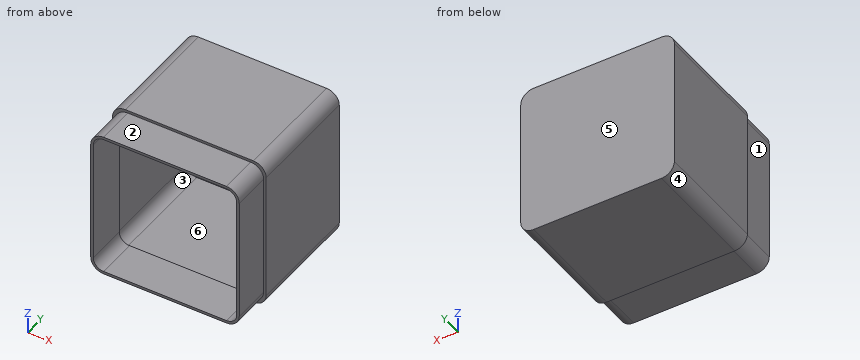
from build123d import *

# Parameters (mm, degrees)
F0_W     = 30.48
F0_H     = 30.48
F1_DEPTH = 22.86
F2_W     = 29.464
F2_H     = 29.464
F3_DEPTH = 7.62
F4_R     = 2.54
F5_T     = -0.508


with BuildPart() as f1:
    # F0 (on Front) → F1 (new body)
    with BuildSketch(Plane.XZ):
        with Locations((15.24, 15.24)):
            Rectangle(F0_W, F0_H)
    extrude(amount=F1_DEPTH)

    # F2 (on face) → F3 (join)
    with BuildSketch(Plane.XZ.offset(22.86)):
        with Locations((15.24, 15.24)):
            Rectangle(F2_W, F2_H)
    extrude(amount=F3_DEPTH)

    # F4
    f4_edges = [f1.edges().sort_by_distance(p)[0] for p in [
        (30.48, -11.43, 30.48),
        (29.972, -26.67, 29.972),
        (0.508, -26.67, 29.972),
        (0, -11.43, 30.48),
        (0, -11.43, 0),
        (0.508, -26.67, 0.508),
        (30.48, -11.43, 0),
        (29.972, -26.67, 0.508),
    ]]
    fillet(f4_edges, radius=F4_R)

    # F5
    f5_openings = [f1.faces().sort_by_distance(p)[0] for p in [
        (15.24, -30.48, 15.24),
    ]]
    offset(amount=F5_T, openings=f5_openings, kind=Kind.INTERSECTION)


solid = f1.part
Geometry check sheet. Reference: the model listing, model coordinates, mm. Face numbers are marked on the shaded views. A direction names the side the tool comes from. Give positions to 0.01 mm unless a question says otherwise; leave off trailing zeros. Write each loop counter-clockwise with the first axis right and the second up, starting at its lowest first coordinate (ties: lowest second). Pieces come first, ordered by that corner, then holes.
1) Release check for a two-part mould opening along Y. For the marked faces 4, 5 and 6 record: released by +Y, released by -Y, zero draft, split by the parting line, or undercut.
Values follow:
face 4: zero draft
face 5: released by +Y
face 6: undercut
2) Cross-section at A-A (z = 14). Record the boundary of the cut face in (x, y).
Values follow:
outline: (0, -22.86) - (0.51, -22.86) - (0.51, -30.48) - (1.02, -30.48) - (1.02, -22.35) - (0.51, -22.35) - (0.51, -0.51) - (29.97, -0.51) - (29.97, -22.35) - (29.46, -22.35) - (29.46, -30.48) - (29.97, -30.48) - (29.97, -22.86) - (30.48, -22.86) - (30.48, 0) - (0, 0) - close
3) Cross-section at C-C (x = 24.5). Record the boundary of the cut face in (y, z), plus the area to 3 significant figures.
Values follow:
outline: (-30.48, 0.51) - (-22.86, 0.51) - (-22.86, 0) - (0, 0) - (0, 30.48) - (-22.86, 30.48) - (-22.86, 29.97) - (-30.48, 29.97) - (-30.48, 29.46) - (-22.35, 29.46) - (-22.35, 29.97) - (-0.51, 29.97) - (-0.51, 0.51) - (-22.35, 0.51) - (-22.35, 1.02) - (-30.48, 1.02) - close
area: 46.5 mm2
4) Thickness scan on line 1 (X direction, y = -3, z = 4.5); line 2 (X direction, y = -24, z = 15.5). Record the ranges inside material, lowest first.
Values follow:
line 1: x = 0 to 0.51, 29.97 to 30.48
line 2: x = 0.51 to 1.02, 29.46 to 29.97
5) Go/stop test with flat-tipped pins: pin 1 Ø2.5 at (y, z) = (-26, 19.5) entering from +X; pin 2 Ø9 at (x, y) = (21, -27.5) entering from +Z; pin 3 Ø9 at (x, z) = (12, 21.5) entering from -Y. Record where each tip stops, or that it passes through.
Values follow:
pin 1: stops at x = 29.97
pin 2: stops at z = 29.97
pin 3: stops at y = -0.51
6) Set-up check for the marked faces 1, 2 and 3: record each of +Z, -Z, +X, -X, +Y, -Y from which the full face is reachable in a straight line by a thin tool's end or side.
Values follow:
face 1: +Z, -Z, -X, -Y
face 2: +Z, +X, -X, -Y
face 3: none
7) Cross-section at B-B (y = -5.5). Record the boundary of the cut face in (x, z), plus the area to 3 significant figures.
Values follow:
outline: (0, 2.54) arc R2.54 ccw to (2.54, 0) - (27.94, 0) arc R2.54 ccw to (30.48, 2.54) - (30.48, 27.94) arc R2.54 ccw to (27.94, 30.48) - (2.54, 30.48) arc R2.54 ccw to (0, 27.94) - close; hole (0.51, 2.54) arc R2.03 ccw to (2.54, 0.51) - (27.94, 0.51) arc R2.03 ccw to (29.97, 2.54) - (29.97, 27.94) arc R2.03 ccw to (27.94, 29.97) - (2.54, 29.97) arc R2.03 ccw to (0.51, 27.94) - close
area: 58.9 mm2
